The listing builds one solid part. Answer for the finished solid, in the listing's coordinates (mm). Face numbers are marked on the shaded views. A direction names the side the tool comes from. Coordinates: 2 decimals unless noted, no trailing zeros. Order: outer loops, then holes, each group sorted by start corner. A loop starts at its lowest first (then second) coordinate and runs counter-clockwise, first axis right, second up.
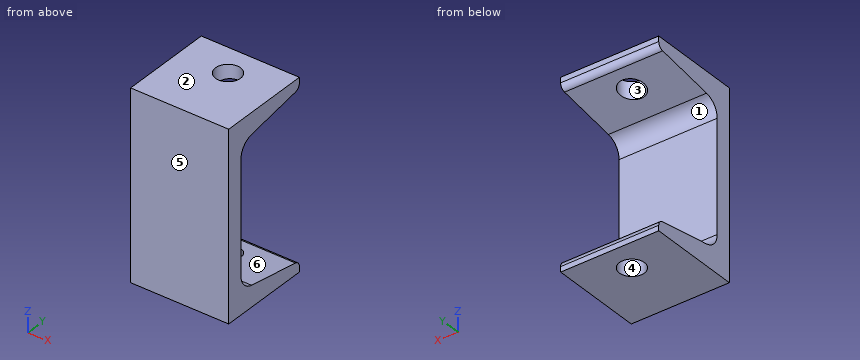
```python
from build123d import *

# Parameters (mm, degrees)
MIEMBRO_ESTRUCTURAL1_DEPTH = 40
CROQUIS4_R                 = 5.1
CORTAR_EXTRUIR1_DEPTH      = 88.834257761


with BuildPart() as part:
    # Sketch1 → Miembro estructural1 (new body)
    with BuildSketch(Plane.YZ.offset(-18.536654135)):
        with BuildLine():
            Line((0, -38.1), (0, 38.1))
            Line((0, 38.1), (38.0492, 38.1))
            Line((38.0492, 38.1), (38.0492, 35.942335136))
            ThreePointArc((38.0492, 35.942335136), (37.447280466, 34.300554363), (35.926803066, 33.436899509))
            Line((35.926803066, 33.436899509), (12.283671721, 29.496090157))
            ThreePointArc((12.283671721, 29.496090157), (8.178382741, 27.164222052), (6.5532, 22.731413966))
            Line((6.5532, 22.731413966), (6.5532, -22.731413966))
            ThreePointArc((6.5532, -22.731413966), (8.178382741, -27.164222052), (12.283671721, -29.496090157))
            Line((12.283671721, -29.496090157), (35.926803066, -33.436899509))
            ThreePointArc((35.926803066, -33.436899509), (37.447280466, -34.300554363), (38.0492, -35.942335136))
            Line((38.0492, -35.942335136), (38.0492, -38.1))
            Line((38.0492, -38.1), (0, -38.1))
        make_face()
    extrude(amount=MIEMBRO_ESTRUCTURAL1_DEPTH)

    # Croquis4 → Cortar-Extruir1 (cut, through all)
    with BuildSketch(Plane.XY.offset(38.1)):
        with Locations((1.463345865, 26.0492)):
            Circle(CROQUIS4_R)
    extrude(amount=-CORTAR_EXTRUIR1_DEPTH, mode=Mode.SUBTRACT)


solid = part.part
```
(1) Find section B-B (y = 14). Write down the section's boundary in (x, z).
(2) The mould has two halves that part along Y. Classify the marked faces 1, 2, 3 and 4: released by +Y, released by -Y, zero draft, split by the parting line, or undercut.
(3) Find section A-A (x = 15.5). Write down the section's boundary in (y, z).
(4) Consider line 1 (Y direction, x = 1, z = -23); line 2 (Z direction, x = 4, y = 33.5); line 3 (Z direction, x = -17, y = 34.5). Determine where each line is inside the solid, lowest interval first.
(5) This flat-tipped pin is pushed along its axis until it touches: pin 1 Ø2 at (x, z) = (-6.5, 27) entering from +Y. Where does it stop, or does it pass through?
(6) Find section C-C (y = 22). Write down the section's boundary in (x, z), and give its area (3 significant figures).
(7) For the marked faces 5 and 6, determine the directions among +Z, -Z, +X, -X, +Y, -Y from which every point of the face is accessible in a straight line to the end or side of a thin tool.
(8) Find section D-D (x = 2). Write down the section's boundary in (y, z), and give its area (3 significant figures).
Findings below:
1. outline: (-18.54, -38.1) - (21.46, -38.1) - (21.46, -29.78) - (-18.54, -29.78) - close; (-18.54, 29.78) - (21.46, 29.78) - (21.46, 38.1) - (-18.54, 38.1) - close
2. face 1: released by +Y
2. face 2: zero draft
2. face 3: undercut
2. face 4: undercut
3. outline: (0, -38.1) - (38.05, -38.1) - (38.05, -35.94) arc R2.54 ccw to (35.93, -33.44) - (12.28, -29.5) arc R6.86 cw to (6.55, -22.73) - (6.55, 22.73) arc R6.86 cw to (12.28, 29.5) - (35.93, 33.44) arc R2.54 ccw to (38.05, 35.94) - (38.05, 38.1) - (0, 38.1) - close
4. line 1: y = 0 to 6.56
4. line 2: z = -38.1 to -33.03, 33.03 to 38.1
4. line 3: z = -38.1 to -33.2, 33.2 to 38.1
5. pin 1: stops at y = 9.02
6. outline: (-18.54, -38.1) - (-1.64, -38.1) - (-1.64, -31.12) - (-18.54, -31.12) - close; (-18.54, 31.12) - (-1.64, 31.12) - (-1.64, 38.1) - (-18.54, 38.1) - close; (4.56, -38.1) - (21.46, -38.1) - (21.46, -31.12) - (4.56, -31.12) - close; (4.56, 31.12) - (21.46, 31.12) - (21.46, 38.1) - (4.56, 38.1) - close
6. area: 472 mm2
7. face 5: +Z, -Z, +X, -X, -Y
7. face 6: +X, -X, +Y
8. outline: (0, -38.1) - (20.98, -38.1) - (20.98, -30.95) - (12.28, -29.5) arc R6.86 cw to (6.55, -22.73) - (6.55, 22.73) arc R6.86 cw to (12.28, 29.5) - (20.98, 30.95) - (20.98, 38.1) - (0, 38.1) - close; (31.12, -38.1) - (38.05, -38.1) - (38.05, -35.94) arc R2.54 ccw to (35.93, -33.44) - (31.12, -32.64) - close; (31.12, 32.64) - (35.93, 33.44) arc R2.54 ccw to (38.05, 35.94) - (38.05, 38.1) - (31.12, 38.1) - close
8. area: 820 mm2
